The listing builds one solid part. Answer for the finished solid, in the listing's coordinates (mm). Coordinates: 2 decimals unless noted, no trailing zeros. Order: outer loops, then holes, each group sorted by start corner. A loop starts at its lowest first (then second) coordinate and runs counter-clockwise, first axis right, second up.
Autodesk Inventor part; units mm, degrees
ref_plane "YZ Plane" through (0, 0, 0) normal (1, 0, 0) x (0, 1, 0)
ref_plane "XZ Plane" through (0, 0, 0) normal (0, 1, 0) x (-1, 0, 0)
ref_plane "XY Plane" through (0, 0, 0) normal (0, 0, 1) x (1, 0, 0)
sketch "Sketch2" plane through (0, 0, 0) normal (0, 0, 1) x (1, 0, 0)
  line L0 (0, 0) -> (-9.9, 0)
  line L1 (-9.9, 0) -> (-9.9, 105)
  line L2 (-9.9, 105) -> (0, 105)
  line L3 (0, 105) -> (0, 0)
  point P0 (-5, 18)
  dimension "d4" = 9.9
  dimension "d5" = 105
extrude "Extrusion2" add sketch "Sketch2" along normal blind 5
sketch "Sketch3" plane through (0, 0, 5) normal (0, 0, 1) x (1, 0, 0)
  point P0 (0, 0)
  point P1 (-4.95, 5)
hole "Hole3" at (-4.95, 5, 5) direction (0, 0, -1) diameter 5 depth 6
properties part number "Elbow_Cube_Holder_TestFit_V2"
1) A cutting plane is placed at C-C, the plane x = -4.95. Write down the section's boundary in (y, z), plus the area to 3 significant figures.
2) A cutting plane is placed at A-A, the plane y = 5. Write down the section's boundary in (x, z).
3) The mould has two halves that part along X. Classify faces 1 (the cylindrical face through (-3.99, 2.69, 2.46)), 2 (the flat face through (-9.9, 52, 2)), 3 (the flat face through (-5, 53, 5)): released by +X, released by -X, zero draft, split by the parting line, or undercut.
4) Straight lines are drawn through the part: probe 1 along X at (y, z) = (5, 3.2); probe 2 along Y at (x, z) = (-4.95, 3.6); probe 3 along Y at (x, z) = (-6.25, 3.1). For each, find the intervals that lie inside material, in ascending order.
5) A cutting plane is placed at B-B, the plane z = 2.95. Write down the section's boundary in (x, y), plus the area to 3 significant figures.
6) Each of these flat-tipped pins is pushed along its axis until it touches: P1, Ø4, axis at x = -4.95, y = 5, coming from the -Z side; P2, Ø4, axis at x = -5.5, y = 80, coming from the -Z side. Where does it stop, or does it pass through?
Working result:
1. outline: (0, 0) - (2.5, 0) - (2.5, 5) - (0, 5) - close; (7.5, 0) - (105, 0) - (105, 5) - (7.5, 5) - close
1. area: 500 mm2
2. outline: (-9.9, 0) - (-7.45, 0) - (-7.45, 5) - (-9.9, 5) - close; (-2.45, 0) - (0, 0) - (0, 5) - (-2.45, 5) - close
3. face 1: undercut
3. face 2: released by -X
3. face 3: zero draft
4. probe 1: x = -9.9 to -7.45, -2.45 to 0
4. probe 2: y = 0 to 2.5, 7.5 to 105
4. probe 3: y = 0 to 2.86, 7.14 to 105
5. outline: (-9.9, 0) - (0, 0) - (0, 105) - (-9.9, 105) - close; hole circle Ø5 at (-4.95, 5)
5. area: 1,020 mm2
6. P1: passes through
6. P2: stops at z = 0
